For this review, use the dimensioned drawing (mm, ordinates from the lowest corner) and the shaded views. Coordinates: 2 decimals unless noted, no trailing zeros. Loops run counter-clockwise (first coordinate to the right, second up) from the corner with the lowest first, then second, coordinate; pieces in that order, holes last. Notation, with made-up numbers: M -40,-23 L 0,-23 A24 cw 0,-12 Z; hole C 89.5,42 d4. An arc over 180 degrees is marked long. Write each question's results on one line, items separated by ' | '. Start each with the question number.
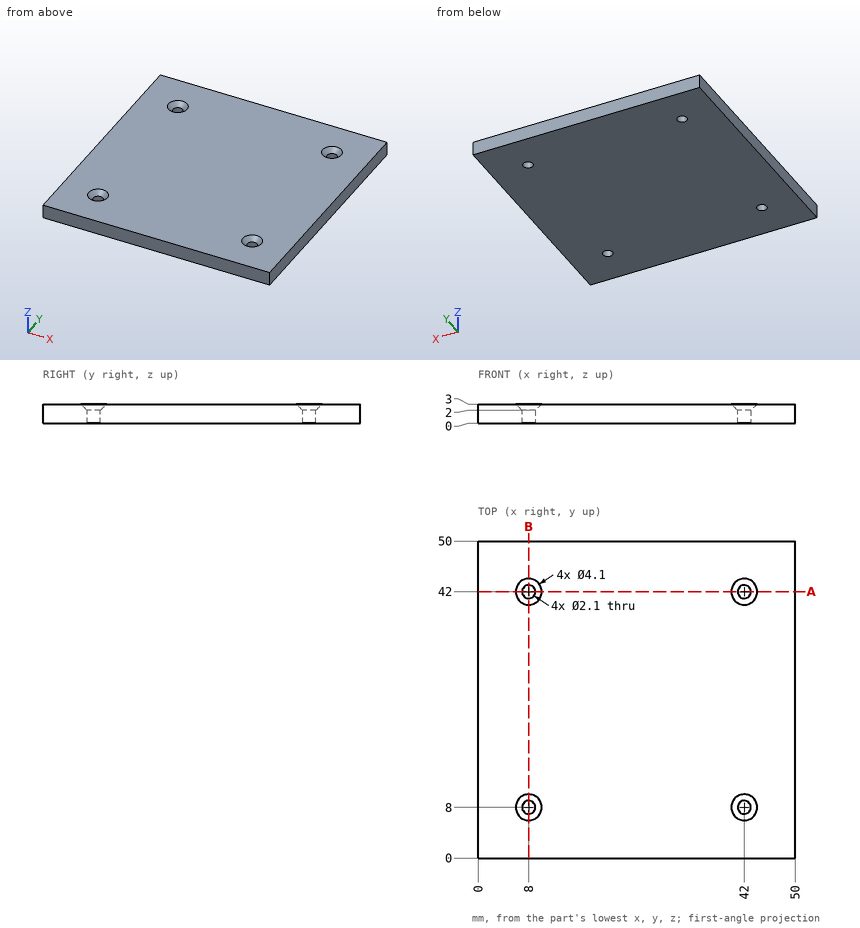
Q1. To check wall thickness, follow line 1 along Y through (x, z) = (42, 0.5); line 2 along X through (y, z) = (9, 2.55). State the ranges of each line that lie inside material, in increasing order.
Q2. Take a section at A-A, the plane y = 42. Give the boundary of the cut face in (x, z), then the cut area to 3 significant figures.
Q3. Insertion check: P1, Ø1.7, axis at x = 42, y = 8, coming from the -Z side; P2, Ø2.5, axis at x = 8, y = 42, coming from the +Z side. Each pin has a flat end and moves straight along its axis. Give the tip position at first contact, or say it passes through.
Results:
1) line 1: 0 to 6.95, 9.05 to 40.95, 43.05 to 50 | line 2: 0 to 6.75, 9.25 to 40.75, 43.25 to 50
2) outline: M 0,0 L 6.95,0 L 6.95,2 L 5.95,3 L 0,3 Z; M 9.05,0 L 40.95,0 L 40.95,2 L 39.95,3 L 10.05,3 L 9.05,2 Z; M 43.05,0 L 50,0 L 50,3 L 44.05,3 L 43.05,2 Z | area: 135 mm^2
3) P1: through | P2: z = 2.2
